Input: part model. Units: mm. Frame: model coordinates. Face numbers are marked on the shaded views. A direction names the side the tool comes from. Give positions to 0.01 mm unless a question says otherwise; leave off trailing zeros. Loops run counter-clockwise (first coordinate to the right, second up) from the corner with the lowest first, then second, coordinate; pieces in that order, holes last. Notation, with made-up numbers: (56, 52) -> (113, 52) arc R13 cw to (113, 65) -> close; hole circle Ø11 at (89.5, -35). An arc over 180 degrees is marked (long way). Answer as a JSON object with one key per item and string values.
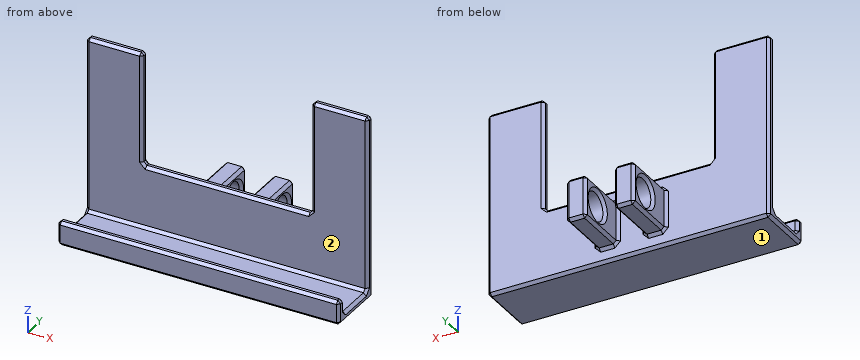
```python
from build123d import *

# Parameters (mm, degrees)
F1_DEPTH = 3
F3_DEPTH = 100
F4_W     = 7
F4_H     = 15
F5_DEPTH = 20
F6_R     = 5
F7_DEPTH = 25
F8_SIZE  = 1


with BuildPart() as f1:
    # F0 (on Front) → F1 (new body)
    with BuildSketch(Plane.XZ):
        Polygon((-48.7427460821, 65), (-48.7427460821, 0), (51.2572539179, 0), (51.2572539179, 65), (31.2572539179, 65), (31.2572539179, 25), (-28.7427460821, 25), (-28.7427460821, 65), align=None)
    extrude(amount=F1_DEPTH)

    # F2 (on face) → F3 (join)
    with BuildSketch(Plane.YZ.offset(51.2572539179)):
        Polygon((-21, 0), (-3, 0), (-3, 2.9999055994), (-18, 2.9999055994), (-18, 8.5), (-21, 8.5), align=None)
    extrude(amount=-F3_DEPTH)

    # F4 (on face) → F5 (join)
    with BuildSketch(Plane(origin=(0, 0, 0), x_dir=(-1, 0, 0), z_dir=(0, 1, 0))):
        with Locations((-8.5, 12.5750002265)):
            Rectangle(F4_W, F4_H)
        with Locations((8.5, 12.5750002265)):
            Rectangle(F4_W, F4_H)
    extrude(amount=F5_DEPTH)

    # F6 (on face) → F7 (cut)
    with BuildSketch(Plane.YZ.offset(12)):
        with Locations((12.5, 12.5750002265)):
            Circle(F6_R)
    extrude(amount=-F7_DEPTH, mode=Mode.SUBTRACT)

    # F8
    f8_edges = [f1.edges().sort_by_distance(p)[0] for p in [
        (1.257254, -3, 2.999906),
        (1.257254, -18, 2.999906),
        (12, 0, 12.575),
        (8.5, 0, 20.075),
        (5, 0, 12.575),
        (8.5, 0, 5.075),
        (-8.5, 0, 5.075),
        (-12, 0, 12.575),
        (-8.5, 0, 20.075),
        (-5, 0, 12.575),
        (12, 7.5, 12.575),
        (5, 7.5, 12.575),
        (-12, 7.5, 12.575),
        (-5, 7.5, 12.575),
        (51.257254, -10.5, 0),
        (1.257254, -21, 0),
        (1.257254, 0, 0),
        (-48.742746, -10.5, 0),
        (1.257254, -21, 8.5),
        (1.257254, -18, 8.5),
        (-48.742746, -19.5, 8.5),
        (51.257254, -19.5, 8.5),
        (1.257254, -3, 25),
        (31.257254, -3, 45),
        (41.257254, -3, 65),
        (51.257254, -3, 33.999953),
        (-48.742746, -3, 33.999953),
        (-48.742746, 0, 32.5),
        (-28.742746, -3, 45),
        (-38.742746, -3, 65),
        (-28.742746, 0, 45),
        (1.257254, 0, 25),
        (31.257254, 0, 45),
        (31.257254, -1.5, 65),
        (31.257254, -1.5, 25),
        (-28.742746, -1.5, 65),
        (51.257254, 0, 32.5),
        (41.257254, 0, 65),
        (-48.742746, -10.5, 2.999906),
        (-38.742746, 0, 65),
        (12, 10, 20.075),
        (5, 10, 20.075),
        (5, 10, 5.075),
        (-5, 10, 20.075),
        (-12, 10, 20.075),
        (-12, 10, 5.075),
        (8.5, 20, 20.075),
        (8.5, 20, 5.075),
        (-5, 20, 12.575),
        (-8.5, 20, 20.075),
        (-12, 20, 12.575),
        (51.257254, -1.5, 65),
        (-28.742746, -1.5, 25),
        (-48.742746, -1.5, 65),
        (-48.742746, -18, 5.749953),
        (51.257254, -10.5, 2.999906),
        (51.257254, -21, 4.25),
        (-48.742746, -21, 4.25),
        (51.257254, -18, 5.749953),
        (12, 20, 12.575),
        (5, 20, 12.575),
        (12, 10, 5.075),
        (-5, 10, 5.075),
        (-8.5, 20, 5.075),
    ]]
    chamfer(f8_edges, length=F8_SIZE)


solid = f1.part
```
Q1. Pin query (flat end, axial travel): pin 1 (16 mm diameter, centred on y = 12.5, z = 12.575, fed in from -X); pin 2 (5 mm diameter, centred on x = -19, y = 1, fed in from +Z); pin 3 (4 mm diameter, centred on x = 8.5, y = 13, fed in from -Z) (3 decimals). Return the tip coordinate at first contact, or that it passes through.
Evaluation:
{"pin 1": "stops at x = -12", "pin 2": "stops at z = 25", "pin 3": "stops at z = 5.075"}
Q2. Section C-C, the plane x = -32.5. Return the cut outline in (y, z), then the cut area to 3 significant figures.
Evaluation:
{"outline": "(-21, 1) -> (-20, 0) -> (-1, 0) -> (0, 1) -> (0, 64) -> (-1, 65) -> (-2, 65) -> (-3, 64) -> (-3, 4) -> (-4, 3) -> (-17, 3) -> (-18, 4) -> (-18, 7.5) -> (-19, 8.5) -> (-20, 8.5) -> (-21, 7.5) -> close", "area": "263 mm2"}
Q3. Section B-B, the plane z = 40. Return the cut outline in (x, y).
Evaluation:
{"outline": "(-48.74, -2) -> (-47.74, -3) -> (-29.74, -3) -> (-28.74, -2) -> (-28.74, -1) -> (-29.74, 0) -> (-47.74, 0) -> (-48.74, -1) -> close; (31.26, -2) -> (32.26, -3) -> (50.26, -3) -> (51.26, -2) -> (51.26, -1) -> (50.26, 0) -> (32.26, 0) -> (31.26, -1) -> close"}
Q4. Access query for the marked faces 1 and 2. Directions: +Z, -Z, +X, -X, +Y, -Y. A direction counts if a zero-diameter tool reaches every point of the face in a straight line with its end or side. Return the directions, or none.
Evaluation:
{"face 1": "-Z, +X, -X, +Y, -Y", "face 2": "+Z, +X, -X"}
Q5. Section A-A, the plane y = 12.5. Give the number of separate pieces and of enclosed holes in the cut face, then the cut area to 3 significant figures.
Evaluation:
{"separate pieces": "4", "enclosed holes": "0", "area": "62.0 mm2"}
Q6. Ray query, line 1 along Z through (x, y) = (8.6, 12.5) (3 decimals); line 2 along Z through (x, y) = (-7, 12) (3 decimals); line 3 along Y through (x, z) = (44.5, 62). Return the intervals inside material, ascending.
Evaluation:
{"line 1": "z = 5.075 to 7.575, 17.575 to 20.075", "line 2": "z = 5.075 to 7.6, 17.55 to 20.075", "line 3": "y = -3 to 0"}
Q7. Section D-D, the plane y = -12. Return the cut outline in (x, z).
Evaluation:
{"outline": "(-48.74, 1) -> (-47.74, 0) -> (50.26, 0) -> (51.26, 1) -> (51.26, 2) -> (50.26, 3) -> (-47.74, 3) -> (-48.74, 2) -> close"}
